```python
from build123d import *

# Parameters (mm, degrees)
SKETCH1_W           = 21.336
SKETCH1_H           = 36.576
SKETCH1_R           = 2.667
BOSS_EXTRUDE1_DEPTH = 1.27


with BuildPart() as part:
    # Sketch1 → Boss-Extrude1 (new body)
    with BuildSketch(Plane(origin=(0, 0, 0), x_dir=(1, 0, 0), z_dir=(0, 1, 0))):
        Rectangle(SKETCH1_W, SKETCH1_H)
        with BuildLine():
            Line((3.018435283, -2.946661255), (2.56364651, -3.401450028))
            ThreePointArc((2.56364651, -3.401450028), (2.768236135, -3.554896302), (2.963662393, -3.719854635))
            ThreePointArc((2.963662393, -3.719854635), (3.148123637, -3.8946201), (3.322296862, -4.079640655))
            ThreePointArc((3.322296862, -4.079640655), (3.486686927, -4.275669436), (3.639526827, -4.480831181))
            Line((3.639526827, -4.480831181), (4.094539809, -4.025818198))
            ThreePointArc((4.094539809, -4.025818198), (4.696624497, -5.096661904), (5.024040768, -6.280727273))
            Line((5.024040768, -6.280727273), (4.380937187, -6.280727273))
            ThreePointArc((4.380937187, -6.280727273), (4.416928537, -6.533901895), (4.438301261, -6.788727273))
            ThreePointArc((4.438301261, -6.788727273), (4.44498858, -7.042743737), (4.437149708, -7.296727273))
            ThreePointArc((4.437149708, -7.296727273), (4.43430089, -7.340889368), (4.431012547, -7.385020912))
            ThreePointArc((4.431012547, -7.385020912), (4.409221171, -7.595511932), (4.377436347, -7.804727273))
            Line((4.377436347, -7.804727273), (5.020988346, -7.804727273))
            ThreePointArc((5.020988346, -7.804727273), (4.691358526, -8.981399356), (4.090276757, -10.045313694))
            Line((4.090276757, -10.045313694), (3.635376444, -9.590413381))
            ThreePointArc((3.635376444, -9.590413381), (3.480018154, -9.798078789), (3.312813037, -9.996330065))
            ThreePointArc((3.312813037, -9.996330065), (3.138047572, -10.180791309), (2.953027016, -10.354964534))
            ThreePointArc((2.953027016, -10.354964534), (2.759829472, -10.51711401), (2.557745709, -10.668044115))
            Line((2.557745709, -10.668044115), (3.012646022, -11.122944428))
            ThreePointArc((3.012646022, -11.122944428), (1.944031836, -11.725975697), (0.762, -12.055192535))
            Line((0.762, -12.055192535), (0.762, -11.411866343))
            ThreePointArc((0.762, -11.411866343), (0.508842492, -11.448446688), (0.254, -11.470404595))
            ThreePointArc((0.254, -11.470404595), (0, -11.477667672), (-0.254, -11.470404595))
            ThreePointArc((-0.254, -11.470404595), (-0.508842492, -11.448446688), (-0.762, -11.411866343))
            Line((-0.762, -11.411866343), (-0.762, -12.055192535))
            ThreePointArc((-0.762, -12.055192535), (-1.944031836, -11.725975697), (-3.012646022, -11.122944428))
            Line((-3.012646022, -11.122944428), (-2.557745709, -10.668044115))
            ThreePointArc((-2.557745709, -10.668044115), (-2.759829472, -10.51711401), (-2.953027016, -10.354964534))
            ThreePointArc((-2.953027016, -10.354964534), (-3.138047572, -10.180791309), (-3.312813037, -9.996330065))
            ThreePointArc((-3.312813037, -9.996330065), (-3.480018154, -9.798078789), (-3.635376444, -9.590413381))
            Line((-3.635376444, -9.590413381), (-4.090276757, -10.045313694))
            ThreePointArc((-4.090276757, -10.045313694), (-4.691358526, -8.981399356), (-5.020988346, -7.804727273))
            Line((-5.020988346, -7.804727273), (-4.377436347, -7.804727273))
            ThreePointArc((-4.377436347, -7.804727273), (-4.414606192, -7.551586906), (-4.437149708, -7.296727273))
            ThreePointArc((-4.437149708, -7.296727273), (-4.44498858, -7.042743737), (-4.438301261, -6.788727273))
            ThreePointArc((-4.438301261, -6.788727273), (-4.416928537, -6.533901895), (-4.380937187, -6.280727273))
            Line((-4.380937187, -6.280727273), (-5.024040768, -6.280727273))
            ThreePointArc((-5.024040768, -6.280727273), (-4.696624497, -5.096661904), (-4.094539809, -4.025818198))
            Line((-4.094539809, -4.025818198), (-3.639526827, -4.480831181))
            ThreePointArc((-3.639526827, -4.480831181), (-3.486686927, -4.275669436), (-3.322296862, -4.079640655))
            ThreePointArc((-3.322296862, -4.079640655), (-3.148123637, -3.8946201), (-2.963662393, -3.719854635))
            ThreePointArc((-2.963662393, -3.719854635), (-2.768236135, -3.554896302), (-2.56364651, -3.401450028))
            Line((-2.56364651, -3.401450028), (-3.018435283, -2.946661255))
            ThreePointArc((-3.018435283, -2.946661255), (-1.94735447, -2.340737305), (-0.762, -2.010142809))
            Line((-0.762, -2.010142809), (-0.762, -2.653469001))
            ThreePointArc((-0.762, -2.653469001), (-0.508842492, -2.616888656), (-0.254, -2.594930748))
            ThreePointArc((-0.254, -2.594930748), (0, -2.587667672), (0.254, -2.594930748))
            ThreePointArc((0.254, -2.594930748), (0.508842492, -2.616888656), (0.762, -2.653469001))
            Line((0.762, -2.653469001), (0.762, -2.010142809))
            ThreePointArc((0.762, -2.010142809), (1.94735447, -2.340737305), (3.018435283, -2.946661255))
        make_face(mode=Mode.SUBTRACT)
        with Locations(Location((0, 11.43, 0), (0, 0, 270))):
            Circle(SKETCH1_R, mode=Mode.SUBTRACT)
    extrude(amount=BOSS_EXTRUDE1_DEPTH)


solid = part.part
```
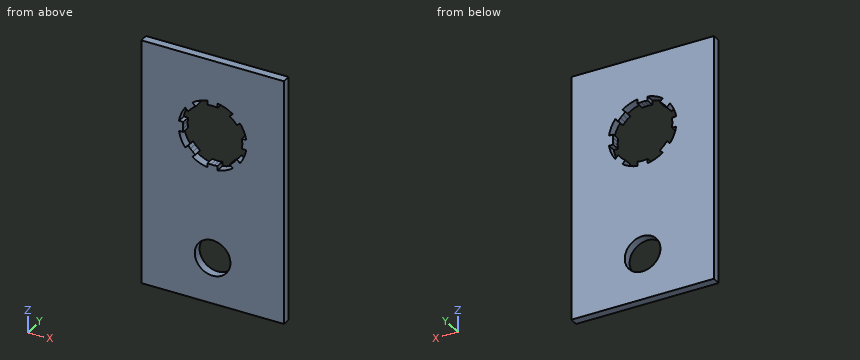
Geometry: final body of the model. Coordinates: model frame, mm. Round coordinates to 2 decimals unless told otherwise and drop trailing zeros. Order: outer loops, then holes, each group sorted by start corner. A loop starts at its lowest first (then second) coordinate and runs counter-clockwise, first axis right, second up. Notation, with made-up numbers: (72.5, 76) - (104.5, 76) arc R33 cw to (104.5, 111) - close; hole circle Ø3 at (69, 42). An arc over 180 degrees is marked (long way). Write item = value, one per line. Start each with the question number.
Q1. Pin query (flat end, axial travel): pin 1 (8 mm diameter, centred on x = 2, z = -7, fed in from -Y); pin 2 (4.5 mm diameter, centred on x = 0, z = -11.43, fed in from +Y). Return the tip coordinate at first contact, or that it passes through.
Q2. Cut plane C-C on y = 0.3. Give the number of separate pieces and of enclosed holes in the cut face, and give its area (3 significant figures).
Q3. Cut plane B-B on x = 1.5. Return the cut outline in (y, z).
Q4. Ray query, line 1 (X direction, y = 1, z = -11.43); line 2 (X direction, y = 1.1, z = 7.5); line 3 (Z direction, x = -2, y = 0.75). Return the intervals inside material, ascending. Write a range as from..to.
Q5. Cut plane A-A on z = -11.43. Return the cut outline in (x, y).
Outcome:
q1.pin_1 = 0
q1.pin_2 = through
q2.separate_pieces = 1
q2.enclosed_holes = 2
q2.area = 685 mm^2
q3.outline = (0, -18.29) - (1.27, -18.29) - (1.27, -13.64) - (0, -13.64) - close; (0, -9.22) - (1.27, -9.22) - (1.27, 2.18) - (0, 2.18) - close; (0, 11.89) - (1.27, 11.89) - (1.27, 18.29) - (0, 18.29) - close
q4.line_1 = -10.67..-2.67, 2.67..10.67
q4.line_2 = -10.67..-4.42, 4.42..10.67
q4.line_3 = -18.29..-13.19, -9.67..2.36, 11.7..18.29
q5.outline = (-10.67, 0) - (-2.67, 0) - (-2.67, 1.27) - (-10.67, 1.27) - close; (2.67, 0) - (10.67, 0) - (10.67, 1.27) - (2.67, 1.27) - close
